Read the model definition and answer for the solid it produces. Units are mm, in the model's axes. A direction names the side the tool comes from. Round coordinates to 2 decimals unless told otherwise and drop trailing zeros. Write each loop counter-clockwise with the first axis right and the second up, starting at its lowest first coordinate (ties: lowest second). Pieces come first, ordered by that corner, then holes. Notation, with made-up numbers: (73, -20.75) - (89, -20.75) arc R18 ccw to (89, 12.25) - close; hole circle Ø8 at (49.25, 20). An arc over 180 degrees is marked (long way). Use one line per item in the form item = value. Start each with the question number.
1) Consider line 1 along Y through (x, z) = (1.5, -2.25); line 2 along X through (y, z) = (-9.5, 0.75); line 3 along X through (y, z) = (6, -0.75). Determine where each line is inside the solid, lowest interval first. Write a range as from..to.
2) The part is cut by section B-B, the plane z = 0. Give the vertices of the cut face in (x, y).
3) The part is cut by section A-A, the plane y = 7.5. Give the vertices of the cut face in (x, z), plus the area to 3 significant figures.
4) The part is cut by section C-C, the plane x = 0. Give the vertices of the cut face in (y, z), plus the area to 3 significant figures.
5) For a pull along Z with two mould halves and no side action, classify faces 4 (the face through (0, -8, -2.36)), 5 (the face through (2.5, 6.8, 0)), 6 (the face through (2.36, -8, 0)) as released by +Z, released by -Z, zero draft, split by the parting line, or undercut.
6) For faces 1 (the face through (0, -8, 2.36)), 2 (the face through (-2, -8, -0.93)), 3 (the face through (-2.5, 6.8, 0)), determine the directions among +Z, -Z, +X, -X, +Y, -Y from which every point of the face is accessible in a straight line to the end or side of a thin tool.
7) Each of these flat-tipped pins is pushed along its axis until it touches: pin 1 (1.6 mm diameter, centred on y = -7, z = -2, fed in from -X); pin 2 (1.6 mm diameter, centred on y = -11, z = 1.5, fed in from +X); pin 3 (1.5 mm diameter, centred on x = 0, y = -11.5, fed in from -Z). Where does it stop, or does it pass through?
8) The part is cut by section D-D, the plane y = 2. Give the vertices of the cut face in (x, z).
from build123d import *

# Parameters (mm, degrees)
F1_DEPTH = 15.72
F2_R     = 5
F3_DEPTH = 10
F5_DEPTH = 6.5


with BuildPart() as f1:
    # F0 (on Front) → F1 (new body)
    with BuildSketch(Plane.XZ):
        Polygon((0.93, 0.93), (0.93, 2.36), (-0.93, 2.36), (-0.93, 0.93), (-2.36, 0.93), (-2.36, -0.93), (-0.93, -0.93), (-0.93, -2.36), (0.93, -2.36), (0.93, -0.93), (2.36, -0.93), (2.36, 0.93), align=None)
    extrude(amount=F1_DEPTH)

    # F2 (on face) → F3 (join)
    with BuildSketch(Plane(origin=(0, 0, 0), x_dir=(-1, 0, 0), z_dir=(0, 1, 0))):
        Circle(F2_R)
    extrude(amount=F3_DEPTH)

    # F4 (on face) → F5 (cut)
    with BuildSketch(Plane(origin=(0, 10, 0), x_dir=(-1, 0, 0), z_dir=(0, 1, 0))):
        with BuildLine():
            ThreePointArc((2, -1.5), (2.5, 0), (2, 1.5))
            Line((2, 1.5), (-2, 1.5))
            ThreePointArc((-2, 1.5), (-2.5, 0), (-2, -1.5))
            Line((-2, -1.5), (2, -1.5))
        make_face()
    extrude(amount=-F5_DEPTH, mode=Mode.SUBTRACT)


solid = f1.part
Geometry results:
q1.line_1 = 0..10
q1.line_2 = -2.36..2.36
q1.line_3 = -4.94..-2.38, 2.38..4.94
q2.outline = (-5, 0) - (-2.36, 0) - (-2.36, -15.72) - (2.36, -15.72) - (2.36, 0) - (5, 0) - (5, 10) - (2.5, 10) - (2.5, 3.5) - (-2.5, 3.5) - (-2.5, 10) - (-5, 10) - close
q3.outline = circle Ø10 at (0, 0); hole (-2, -1.5) - (2, -1.5) arc R2.5 ccw to (2, 1.5) - (-2, 1.5) arc R2.5 ccw to start
q3.area = 64.5 mm2
q4.outline = (-15.72, -2.36) - (0, -2.36) - (0, -5) - (10, -5) - (10, -1.5) - (3.5, -1.5) - (3.5, 1.5) - (10, 1.5) - (10, 5) - (0, 5) - (0, 2.36) - (-15.72, 2.36) - close
q4.area = 155 mm2
q5.face_4 = released by -Z
q5.face_5 = undercut
q5.face_6 = zero draft
q6.face_1 = +Z, +X, -X, -Y
q6.face_2 = -Z, -X, -Y
q6.face_3 = +Y
q7.pin_1 = -0.93
q7.pin_2 = 2.36
q7.pin_3 = -2.36
q8.outline = circle Ø10 at (0, 0)
